from build123d import *

# Parameters (mm, degrees)
SKETCH2_W                 = 30
SKETCH2_H                 = 22
BASE_FLANGE1_DEPTH        = 2
EDGE_FLANGE1_START        = -11
EDGE_FLANGE1_DEPTH        = 22
EDGE_FLANGE1_2_DEPTH      = 22
F_6_0MM_DOWEL_HOLE1_D     = 6
F_6_0MM_DOWEL_HOLE1_DEPTH = 2
F_3_0MM_DOWEL_HOLE1_D     = 3


# Read off the part's stored shape, not the designer's step: Edge-Flange1
# Sheet-metal steps are written as plain solids
with BuildPart() as part:
    # Sketch2 → Base-Flange1 (new body)
    with BuildSketch(Plane(origin=(0, 0, 0), x_dir=(1, 0, 0), z_dir=(0, 1, 0))):
        with Locations((-15, 0)):
            Rectangle(SKETCH2_W, SKETCH2_H)
    extrude(amount=-BASE_FLANGE1_DEPTH)

    # Edge-Flange1 outline → Edge-Flange1 (cut)
    with BuildSketch(Plane.XY.offset(EDGE_FLANGE1_START)):
        with BuildLine():
            ThreePointArc((-26.96949183, -2), (-28.62375904, -1.443395312), (-29.605094228, 0))
            Line((-29.605094228, 0), (-30, 0))
            Line((-30, 0), (-30, -2))
            Line((-30, -2), (-26.96949183, -2))
        make_face()
    extrude(amount=EDGE_FLANGE1_DEPTH, mode=Mode.SUBTRACT)

    # Edge-Flange1 2 outline → Edge-Flange1 2 (add)
    with BuildSketch(Plane.XY.offset(EDGE_FLANGE1_START)):
        with BuildLine():
            Line((-2.065803424, 104.251840892), (-29.612844446, 1.444884199))
            ThreePointArc((-29.612844446, 1.444884199), (-29.706052463, 0.721921355), (-29.605094228, 0))
            Line((-29.605094228, 0), (-26.96949183, 0))
            ThreePointArc((-26.96949183, 0), (-27.5538759, 0.288186332), (-27.680992793, 0.927246109))
            Line((-27.680992793, 0.927246109), (-0.133951771, 103.734202802))
            Line((-0.133951771, 103.734202802), (-2.065803424, 104.251840892))
        make_face()
    extrude(amount=EDGE_FLANGE1_2_DEPTH)

    # Ø6.0mm Dowel Hole1
    with Locations(Plane(origin=(0, 0, 0), x_dir=(1, 0, 0), z_dir=(0, 1, 0))):
        with Locations((-8, 0)):
            Hole(F_6_0MM_DOWEL_HOLE1_D / 2, depth=F_6_0MM_DOWEL_HOLE1_DEPTH)

    # Ø3.0mm Dowel Hole1 (through all)
    with Locations(Plane(origin=(-27.990381057, 7.5, 0), x_dir=(0, 0, 1), z_dir=(-0.9659258262890691, 0.258819045102518, 0))):
        with Locations((0, 85.764876286), (0, 36.764876286)):
            Hole(F_3_0MM_DOWEL_HOLE1_D / 2)


solid = part.part
Here's how the part is built. I have some questions about the finished solid (model axes, mm). A direction names the side the tool comes from. Give positions to 0.01 mm unless a question says otherwise; leave off trailing zeros. Loops run counter-clockwise (first coordinate to the right, second up) from the corner with the lowest first, then second, coordinate; pieces in that order, holes last. Notation, with made-up numbers: (-8, 62.25) -> (6, 62.25) arc R29 ccw to (6, 83.25) -> close; hole circle Ø4 at (20, 73). An arc over 180 degrees is marked (long way). One line per item, written item: value.
Q1. We'd pull the mould along X, two halves only. Please class faces 3 (the face through (-10.77, -1.01, 1.15)), 4 (the face through (-14, -2, 0)), 5 (the face through (-15.646, 53.568, -0.154)), 6 (the face through (0, -1, 0)): pulls with the +X half, pulls with the -X half, needs draft (parallel to the pull), parting line crosses it, or undercut.
Answers follow:
face 3: undercut
face 4: needs draft
face 5: pulls with the -X half
face 6: pulls with the +X half
Q2. Suppose I cut it at A-A on x = -24. Please give me the cut outline in (y, z).
Answers follow:
outline: (-2, -11) -> (0, -11) -> (0, 11) -> (-2, 11) -> close; (14.66, -11) -> (22.39, -11) -> (22.39, 11) -> (14.66, 11) -> close
Q3. Suppose I cut it at C-C on x = -8. Please give me the cut outline in (y, z), then the cut area to 3 significant figures.
Answers follow:
outline: (-2, -11) -> (0, -11) -> (0, -3) -> (-2, -3) -> close; (-2, 3) -> (0, 3) -> (0, 11) -> (-2, 11) -> close; (74.38, -11) -> (82.11, -11) -> (82.11, 11) -> (74.38, 11) -> close
area: 202 mm^2
Q4. On a 3-axis mill with a long thin cutter (end or side, diameter ignored), from which of +Z, -Z, +X, -X, +Y, -Y can I reach the whole of each face in a straight line? I mean faces 1 (the face through (-14.1, 51.61, -0.15)), 2 (the face through (-5, 89.2, 1.2)). Say none if no direction works.
Answers follow:
face 1: +Z, -Z, +X
face 2: none
Q5. I'm going to push flat-ended pins straight in: pin 1 Ø10 at (x, y) = (-20, 67) entering from +Z; pin 2 Ø10 at (x, z) = (-3, 5) entering from +Y; pin 3 Ø5 at (y, z) = (38.5, -3) entering from +X; pin 4 Ø10 at (y, z) = (93.5, 7.5) entering from +X. Where does each tip first touch, or does it pass through?
Answers follow:
pin 1: through
pin 2: y = 104.25
pin 3: x = -16.94
pin 4: x = -1.54
Q6. Suppose I cut it at D-D on y = 52.5. Please give me the cut outline in (x, z).
Answers follow:
outline: (-15.93, -11) -> (-13.86, -11) -> (-13.86, 11) -> (-15.93, 11) -> close
Q7. Suppose I cut it at B-B on z = 0. Please give me the cut outline in (x, y).
Answers follow:
outline: (-29.61, 1.44) arc R2.74 ccw to (-26.97, -2) -> (-11, -2) -> (-11, 0) -> (-26.97, 0) arc R0.74 cw to (-27.68, 0.93) -> (-16.93, 41.05) -> (-18.86, 41.56) -> close; (-18.09, 44.46) -> (-16.15, 43.94) -> (-4.25, 88.38) -> (-6.18, 88.89) -> close; (-5.4, 91.79) -> (-3.47, 91.27) -> (-0.13, 103.73) -> (-2.07, 104.25) -> close; (-5, -2) -> (0, -2) -> (0, 0) -> (-5, 0) -> close
Q8. If I drill on line 1 along Z through (x, y) = (-8, -0.35); line 2 along X through (y, z) = (8.5, 6.25); line 3 along X through (y, z) = (34.5, -5.75), over which ranges is the centre line in solid material (lowest first)?
Answers follow:
line 1: -11 to -3, 3 to 11
line 2: -27.72 to -25.65
line 3: -20.76 to -18.69
